from build123d import *

# Parameters (mm, degrees)
F1_DEPTH = 1.2
F3_DEPTH = 0.2


with BuildPart() as f1:
    # F0 (on Top) → F1 (new body)
    with BuildSketch(Plane.XY):
        Polygon((-4.5237019658, 9.4786183909), (-13.8142090873, 9.4786183909), (-13.8142090873, -9.2292996123), (6.1857909127, -9.2292996123), (6.1857909127, 3.2034474425), (15.4762980342, 3.2034474425), (15.4762980342, 18.2034474425), (-4.5237019658, 18.2034474425), align=None)
        Polygon((-4.1237018444, 9.0786182694), (-4.1237018444, 17.8034473211), (15.0762979127, 17.8034473211), (15.0762979127, 3.6034475639), (5.7857907913, 3.6034475639), (5.7857907913, -8.8292994909), (-13.4142089658, -8.8292994909), (-13.4142089658, 9.0786182694), align=None, mode=Mode.SUBTRACT)
    extrude(amount=F1_DEPTH)

    # F2 (on face) → F3 (join)
    with BuildSketch(Plane(origin=(0, 0, 0), x_dir=(1, 0, 0), z_dir=(0, 0, -1))):
        with BuildLine():
            Line((-13.4142089658, 8.8292994909), (-11.4142089658, 8.8292994909))
            ThreePointArc((-11.4142089658, 8.8292994909), (-11.4243366661, 9.0303174766), (-11.4546171964, 9.2292996123))
            Line((-11.4546171964, 9.2292996123), (-13.8142090873, 9.2292996123))
            Line((-13.8142090873, 9.2292996123), (-13.8142090873, 6.8697077215))
            ThreePointArc((-13.8142090873, 6.8697077215), (-13.6152269515, 6.8394271911), (-13.4142089658, 6.8292994909))
            Line((-13.4142089658, 6.8292994909), (-13.4142089658, 8.8292994909))
        make_face()
        with BuildLine():
            ThreePointArc((-13.4142089658, 6.8292994909), (-11.9999954035, 7.4150859285), (-11.4142089658, 8.8292994909))
            Line((-11.4142089658, 8.8292994909), (-13.4142089658, 8.8292994909))
            Line((-13.4142089658, 8.8292994909), (-13.4142089658, 6.8292994909))
        make_face()
        with BuildLine():
            Line((-13.8142090873, 9.2292996123), (-11.4546171964, 9.2292996123))
            ThreePointArc((-11.4546171964, 9.2292996123), (-14.8284225282, 10.2435130533), (-13.8142090873, 6.8697077215))
            Line((-13.8142090873, 6.8697077215), (-13.8142090873, 9.2292996123))
        make_face()
        with BuildLine():
            Line((5.7857907913, 8.8292994909), (4.2261991433, 8.8292994909))
            ThreePointArc((4.2261991433, 8.8292994909), (4.7715773503, 7.81508605), (5.7857907913, 7.2697078429))
            Line((5.7857907913, 7.2697078429), (5.7857907913, 8.8292994909))
        make_face()
        with BuildLine():
            ThreePointArc((4.1857909127, 9.2292996123), (4.1959186129, 9.0282816267), (4.2261991433, 8.8292994909))
            Line((4.2261991433, 8.8292994909), (5.7857907913, 8.8292994909))
            Line((5.7857907913, 8.8292994909), (5.7857907913, 7.2697078429))
            ThreePointArc((5.7857907913, 7.2697078429), (5.984772927, 7.2394273126), (6.1857909127, 7.2292996123))
            Line((6.1857909127, 7.2292996123), (6.1857909127, 9.2292996123))
            Line((6.1857909127, 9.2292996123), (4.1857909127, 9.2292996123))
        make_face()
        with BuildLine():
            ThreePointArc((8.1857909127, 9.2292996123), (6.1857909127, 11.2292996123), (4.1857909127, 9.2292996123))
            Line((4.1857909127, 9.2292996123), (6.1857909127, 9.2292996123))
            Line((6.1857909127, 9.2292996123), (6.1857909127, 7.2292996123))
            ThreePointArc((6.1857909127, 7.2292996123), (7.6000044751, 7.81508605), (8.1857909127, 9.2292996123))
        make_face()
        with BuildLine():
            Line((-13.8142090873, -9.4786183909), (-13.8142090873, -7.4786183909))
            ThreePointArc((-13.8142090873, -7.4786183909), (-15.2284226497, -10.8928319532), (-11.8142090873, -9.4786183909))
            Line((-11.8142090873, -9.4786183909), (-13.8142090873, -9.4786183909))
        make_face()
        with BuildLine():
            Line((-13.4142089658, -9.0786182694), (-13.4142089658, -7.5190266214))
            ThreePointArc((-13.4142089658, -7.5190266214), (-13.6131911016, -7.4887460911), (-13.8142090873, -7.4786183909))
            Line((-13.8142090873, -7.4786183909), (-13.8142090873, -9.4786183909))
            Line((-13.8142090873, -9.4786183909), (-11.8142090873, -9.4786183909))
            ThreePointArc((-11.8142090873, -9.4786183909), (-11.8243367875, -9.2776004052), (-11.8546173178, -9.0786182694))
            Line((-11.8546173178, -9.0786182694), (-13.4142089658, -9.0786182694))
        make_face()
        with BuildLine():
            ThreePointArc((-11.8546173178, -9.0786182694), (-12.3999955249, -8.0644048285), (-13.4142089658, -7.5190266214))
            Line((-13.4142089658, -7.5190266214), (-13.4142089658, -9.0786182694))
            Line((-13.4142089658, -9.0786182694), (-11.8546173178, -9.0786182694))
        make_face()
        with BuildLine():
            ThreePointArc((-2.1237018444, -9.0786182694), (-4.1237018444, -7.0786182694), (-6.1237018444, -9.0786182694))
            Line((-6.1237018444, -9.0786182694), (-4.1237018444, -9.0786182694))
            Line((-4.1237018444, -9.0786182694), (-4.1237018444, -11.0786182694))
            ThreePointArc((-4.1237018444, -11.0786182694), (-2.709488282, -10.4928318318), (-2.1237018444, -9.0786182694))
        make_face()
        with BuildLine():
            Line((-4.1237018444, -9.0786182694), (-6.1237018444, -9.0786182694))
            ThreePointArc((-6.1237018444, -9.0786182694), (-6.1135741441, -9.2796362551), (-6.0832936138, -9.4786183909))
            Line((-6.0832936138, -9.4786183909), (-4.5237019658, -9.4786183909))
            Line((-4.5237019658, -9.4786183909), (-4.5237019658, -11.0382100389))
            ThreePointArc((-4.5237019658, -11.0382100389), (-4.32471983, -11.0684905692), (-4.1237018444, -11.0786182694))
            Line((-4.1237018444, -11.0786182694), (-4.1237018444, -9.0786182694))
        make_face()
        with BuildLine():
            Line((-4.5237019658, -9.4786183909), (-6.0832936138, -9.4786183909))
            ThreePointArc((-6.0832936138, -9.4786183909), (-5.5379154067, -10.4928318318), (-4.5237019658, -11.0382100389))
            Line((-4.5237019658, -11.0382100389), (-4.5237019658, -9.4786183909))
        make_face()
        with BuildLine():
            ThreePointArc((-2.1237018444, -17.8034473211), (-2.709488282, -16.3892337587), (-4.1237018444, -15.8034473211))
            Line((-4.1237018444, -15.8034473211), (-4.1237018444, -17.8034473211))
            Line((-4.1237018444, -17.8034473211), (-2.1237018444, -17.8034473211))
        make_face()
        with BuildLine():
            ThreePointArc((-4.1237018444, -15.8034473211), (-4.32471983, -15.8135750213), (-4.5237019658, -15.8438555516))
            Line((-4.5237019658, -15.8438555516), (-4.5237019658, -18.2034474425))
            Line((-4.5237019658, -18.2034474425), (-2.1641100749, -18.2034474425))
            ThreePointArc((-2.1641100749, -18.2034474425), (-2.1338295446, -18.0044653067), (-2.1237018444, -17.8034473211))
            Line((-2.1237018444, -17.8034473211), (-4.1237018444, -17.8034473211))
            Line((-4.1237018444, -17.8034473211), (-4.1237018444, -15.8034473211))
        make_face()
        with BuildLine():
            Line((-4.5237019658, -18.2034474425), (-4.5237019658, -15.8438555516))
            ThreePointArc((-4.5237019658, -15.8438555516), (-5.5379154067, -19.2176608834), (-2.1641100749, -18.2034474425))
            Line((-2.1641100749, -18.2034474425), (-4.5237019658, -18.2034474425))
        make_face()
        with BuildLine():
            Line((15.0762979127, -17.8034473211), (15.0762979127, -15.8034473211))
            ThreePointArc((15.0762979127, -15.8034473211), (13.6620843504, -16.3892337587), (13.0762979127, -17.8034473211))
            Line((13.0762979127, -17.8034473211), (15.0762979127, -17.8034473211))
        make_face()
        with BuildLine():
            ThreePointArc((15.4762980342, -15.8438555516), (15.2773158984, -15.8135750213), (15.0762979127, -15.8034473211))
            Line((15.0762979127, -15.8034473211), (15.0762979127, -17.8034473211))
            Line((15.0762979127, -17.8034473211), (13.0762979127, -17.8034473211))
            ThreePointArc((13.0762979127, -17.8034473211), (13.086425613, -18.0044653067), (13.1167061433, -18.2034474425))
            Line((13.1167061433, -18.2034474425), (15.4762980342, -18.2034474425))
            Line((15.4762980342, -18.2034474425), (15.4762980342, -15.8438555516))
        make_face()
        with BuildLine():
            ThreePointArc((17.0762979127, -17.8034473211), (16.6254912904, -16.538536305), (15.4762980342, -15.8438555516))
            Line((15.4762980342, -15.8438555516), (15.4762980342, -18.2034474425))
            Line((15.4762980342, -18.2034474425), (13.1167061433, -18.2034474425))
            ThreePointArc((13.1167061433, -18.2034474425), (15.2773158984, -19.7933196208), (17.0762979127, -17.8034473211))
        make_face()
        with BuildLine():
            ThreePointArc((17.0762979127, -3.6034475639), (15.2773158984, -1.6135752642), (13.1167061433, -3.2034474425))
            Line((13.1167061433, -3.2034474425), (15.4762980342, -3.2034474425))
            Line((15.4762980342, -3.2034474425), (15.4762980342, -5.5630393334))
            ThreePointArc((15.4762980342, -5.5630393334), (16.6254912904, -4.86835858), (17.0762979127, -3.6034475639))
        make_face()
        with BuildLine():
            ThreePointArc((13.1167061433, -3.2034474425), (13.086425613, -3.4024295783), (13.0762979127, -3.6034475639))
            Line((13.0762979127, -3.6034475639), (15.0762979127, -3.6034475639))
            Line((15.0762979127, -3.6034475639), (15.0762979127, -5.6034475639))
            ThreePointArc((15.0762979127, -5.6034475639), (15.2773158984, -5.5933198637), (15.4762980342, -5.5630393334))
            Line((15.4762980342, -5.5630393334), (15.4762980342, -3.2034474425))
            Line((15.4762980342, -3.2034474425), (13.1167061433, -3.2034474425))
        make_face()
        with BuildLine():
            Line((15.0762979127, -3.6034475639), (13.0762979127, -3.6034475639))
            ThreePointArc((13.0762979127, -3.6034475639), (13.6620843504, -5.0176611263), (15.0762979127, -5.6034475639))
            Line((15.0762979127, -5.6034475639), (15.0762979127, -3.6034475639))
        make_face()
        with BuildLine():
            Line((5.7857907913, -3.6034475639), (5.7857907913, -1.6034475639))
            ThreePointArc((5.7857907913, -1.6034475639), (4.3715772289, -5.0176611263), (7.7857907913, -3.6034475639))
            Line((7.7857907913, -3.6034475639), (5.7857907913, -3.6034475639))
        make_face()
        with BuildLine():
            ThreePointArc((6.1857909127, -1.6438557945), (5.9868087769, -1.6135752642), (5.7857907913, -1.6034475639))
            Line((5.7857907913, -1.6034475639), (5.7857907913, -3.6034475639))
            Line((5.7857907913, -3.6034475639), (7.7857907913, -3.6034475639))
            ThreePointArc((7.7857907913, -3.6034475639), (7.7756630911, -3.4024295783), (7.7453825607, -3.2034474425))
            Line((7.7453825607, -3.2034474425), (6.1857909127, -3.2034474425))
            Line((6.1857909127, -3.2034474425), (6.1857909127, -1.6438557945))
        make_face()
        with BuildLine():
            ThreePointArc((7.7453825607, -3.2034474425), (7.2000043536, -2.1892340016), (6.1857909127, -1.6438557945))
            Line((6.1857909127, -1.6438557945), (6.1857909127, -3.2034474425))
            Line((6.1857909127, -3.2034474425), (7.7453825607, -3.2034474425))
        make_face()
    extrude(amount=-F3_DEPTH)


solid = f1.part
For this review, take the finished solid that the model builds, in its own axes (mm). A direction names the side the tool comes from. Coordinates: 2 decimals unless noted, no trailing zeros. Write each loop counter-clockwise with the first axis right and the second up, starting at its lowest first coordinate (ties: lowest second). Pieces come first, ordered by that corner, then holes. Notation, with made-up numbers: (37.5, 18) -> (43.5, 18) arc R13 ccw to (43.5, 34) -> close; hole circle Ø11 at (-17, 26.25). An arc over 180 degrees is marked (long way). Write each question's results on one line, items separated by ' | '. Start each with the question number.
1) The part is to be moulded in two halves that separate along Y. For faces 4 (the face through (6, 18.203, 1)), 5 (the face through (-4, -9.229, 1)), 6 (the face through (-4, -8.829, 1)), say which applies: +Y half, -Y half, draft (parallel to the pull), parting line (faces both ways), or undercut.
2) Consider section C-C (z = 0.65). Write out the cut boundary in (x, y), plus the area to 3 significant figures.
3) Consider section B-B (y = 13). Write out the cut boundary in (x, z), plus the area to 3 significant figures.
4) Consider section D-D (x = -3.5). Write out the cut boundary in (y, z), plus the area to 3 significant figures.
5) Consider section A-A (x = -11). Write out the cut boundary in (y, z), plus the area to 3 significant figures.
6) For faces 1 (the face through (-13, 8, 0.2)), 2 (the face through (4, 4, 0)), 3 (the face through (7, 3, 0.2)), list the 3-axis set-ups (+Z, -Z, +X, -X, +Y, -Y) from which the entire face can be reached by the end or side of a thin tool; tool diameter is ignored.
7) Wall thickness on L1, parallel to Y at x = -3.5, z = 0.25; L2, parallel to X at y = -1.5, z = 1.05; L3, parallel to Y at x = -9.5, z = 0.1: over which ranges is each line inside the solid? List them lowest first. Write a range as [from, to].
8) Insertion check: pin 1 (5 mm diameter, centred on x = -12, y = 4.5, fed in from -Z); pin 2 (0.6 mm diameter, centred on x = 3, z = 0.5, fed in from +Y); pin 3 (2 mm diameter, centred on x = 3, y = 15.5, fed in from +Z); pin 4 (0.6 mm diameter, centred on y = 12.5, z = 1, fed in from -X). Each pin has a flat end and moves straight along its axis. Give the tip position at first contact, or say it passes through.
Geometry says:
1) face 4: +Y half | face 5: -Y half | face 6: undercut
2) outline: (-13.81, -9.23) -> (6.19, -9.23) -> (6.19, 3.2) -> (15.48, 3.2) -> (15.48, 18.2) -> (-4.52, 18.2) -> (-4.52, 9.48) -> (-13.81, 9.48) -> close; hole (-13.41, -8.83) -> (5.79, -8.83) -> (5.79, 3.6) -> (15.08, 3.6) -> (15.08, 17.8) -> (-4.12, 17.8) -> (-4.12, 9.08) -> (-13.41, 9.08) -> close | area: 44.7 mm^2
3) outline: (-4.52, 0) -> (-4.12, 0) -> (-4.12, 1.2) -> (-4.52, 1.2) -> close; (15.08, 0) -> (15.48, 0) -> (15.48, 1.2) -> (15.08, 1.2) -> close | area: 0.960 mm^2
4) outline: (-9.23, 0) -> (-8.83, 0) -> (-8.83, 1.2) -> (-9.23, 1.2) -> close; (7.18, 0) -> (10.98, 0) -> (10.98, 0.2) -> (7.18, 0.2) -> close; (15.9, 0) -> (19.7, 0) -> (19.7, 0.2) -> (18.2, 0.2) -> (18.2, 1.2) -> (17.8, 1.2) -> (17.8, 0.2) -> (15.9, 0.2) -> close | area: 2.40 mm^2
5) outline: (-9.23, 0) -> (-8.83, 0) -> (-8.83, 1.2) -> (-9.23, 1.2) -> close; (9.08, 0) -> (9.48, 0) -> (9.48, 1.2) -> (9.08, 1.2) -> close | area: 0.960 mm^2
6) face 1: +Z | face 2: -Z, +X, -X, +Y, -Y | face 3: +Z, +X, -Y
7) L1: [-9.23, -8.83], [17.8, 18.2] | L2: [-13.81, -13.41], [5.79, 6.19] | L3: [-9.23, -8.83], [9.08, 9.48]
8) pin 1: z = 0 | pin 2: y = 18.2 | pin 3: through | pin 4: x = -4.52
